Input: dimensioned drawing with shaded views. Units: mm. Origin: part minimum x, y, z. A direction names the side the tool comes from. Coordinates: 2 decimals unless noted, no trailing zeros. Order: outer loops, then holes, each group sorted by start corner. A loop starts at its lowest first (then second) coordinate and runs counter-clockwise, first axis right, second up.
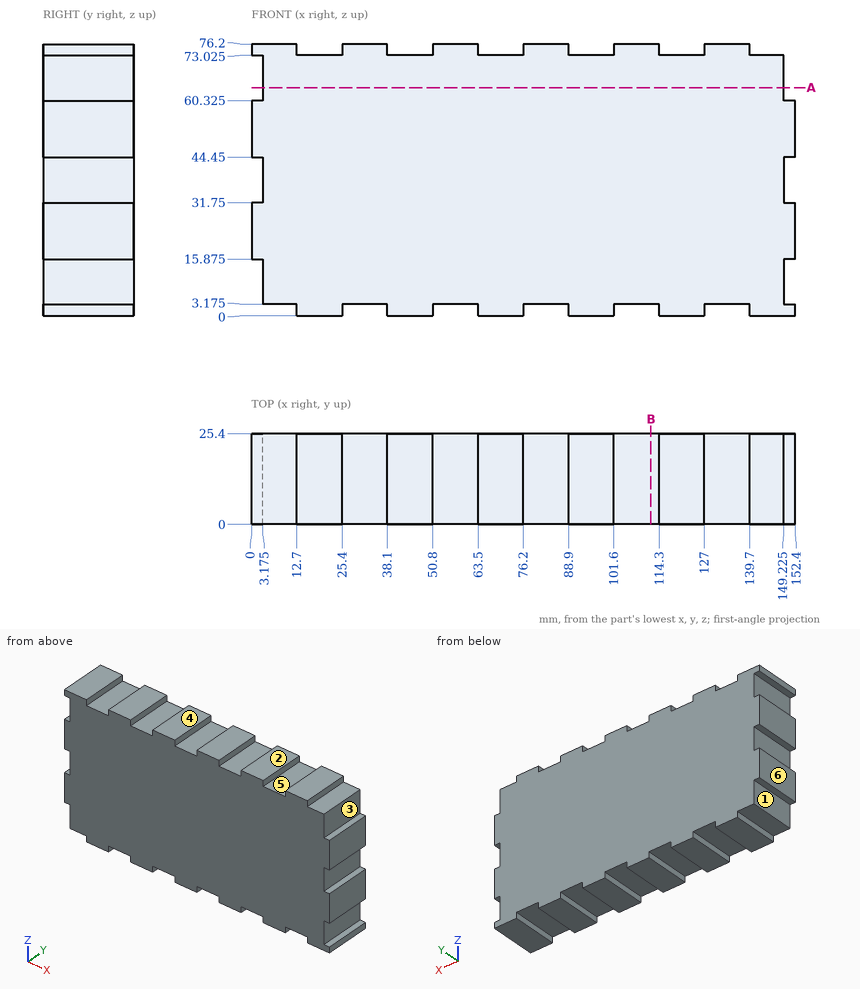
1. Section query B-B on x = 112. Return loops of the section in (y, z) (3 decimals), plus the area to 3 significant figures.
Findings:
outline: (0, 3.175) - (25.4, 3.175) - (25.4, 76.2) - (0, 76.2) - close
area: 1,850 mm2
2. Section query A-A on z = 64. Return loops of the section in (x, y) (3 decimals).
Findings:
outline: (3.175, 0) - (149.225, 0) - (149.225, 25.4) - (3.175, 25.4) - close
3. Draft query along X for the marked faces 4, 5 and 6. Return one class per face: released by +X, released by -X, zero draft, split by the parting line, or undercut.
Findings:
face 4: zero draft
face 5: undercut
face 6: released by -X
4. Pin query (flat end, axial travel): P1, Ø3.5, axis at y = 16, z = 1.5, coming from the -X side (3 decimals); P2, Ø1.6, axis at x = 151.5, y = 11, coming from the +Z side (3 decimals); P3, Ø1, axis at y = 16, z = 1.5, coming from the -X side. Return the tip coordinate at first contact, or that it passes through.
Findings:
P1: stops at x = 3.175
P2: stops at z = 60.325
P3: stops at x = 12.7
5. Ray query, line 1 (X direction, y = 10.25, z = 69) (3 decimals); line 2 (Z direction, x = 33, y = 24.75) (3 decimals); line 3 (Z direction, x = 120.5, y = 4.25) (3 decimals). Return the intervals inside material, ascending.
Findings:
line 1: x = 3.175 to 149.225
line 2: z = 3.175 to 76.2
line 3: z = 0 to 73.025
6. Access query for the marked faces 1, 2 and 3. Directions: +Z, -Z, +X, -X, +Y, -Y. A direction counts if a zero-diameter tool reaches every point of the face in a straight line with its end or side. Return the directions, or none.
Findings:
face 1: -Z, -X, +Y, -Y
face 2: +Z, +X, -X, +Y, -Y
face 3: +Z, +X, +Y, -Y
